```python
from build123d import *

# Parameters (mm, degrees)
SASE_TABAN1_W               = 80
SASE_TABAN1_H               = 130
Y_KSEKLIK_EKSTR_ZYON4_DEPTH = 3
SASE_TABAN1_5_W             = 86
SASE_TABAN1_5_H             = 136
SASE_TABAN1_5_W_2           = 80
SASE_TABAN1_5_H_2           = 130
Y_KSEKLIK_EKSTR_ZYON5_DEPTH = 10
Y_KSEKLIK_EKSTR_ZYON6_REACH = 138.755
KES_EKSTR_ZYON1_START       = -13
EKLEM_ORTA_W                = 36
EKLEM_ORTA_H                = 15
KES_EKSTR_ZYON1_DEPTH       = 13
KES_EKSTR_ZYON3_DEPTH       = 42
KES_EKSTR_ZYON4_START       = -6
KES_EKSTR_ZYON4_DEPTH       = 6
Y_KSEKLIK_EKSTR_ZYON7_START = -3
Y_KSEKLIK_EKSTR_ZYON7_DEPTH = 3
Y_KSEKLIK_EKSTR_ZYON8_DEPTH = 3


with BuildPart() as part:
    # sase_taban1 → Yükseklik-Ekstrüzyon4 (new body)
    with BuildSketch(Plane.XY):
        with Locations((1.981566113, 37.857486255)):
            Rectangle(SASE_TABAN1_W, SASE_TABAN1_H)
    extrude(amount=-Y_KSEKLIK_EKSTR_ZYON4_DEPTH)

    # sase_taban1<5> → Yükseklik-Ekstrüzyon5 (add)
    with BuildSketch(Plane.XY):
        with Locations((1.981566113, 37.857486255)):
            Rectangle(SASE_TABAN1_5_W, SASE_TABAN1_5_H)
        with Locations((1.981566113, 37.857486255)):
            Rectangle(SASE_TABAN1_5_W_2, SASE_TABAN1_5_H_2, mode=Mode.SUBTRACT)
    extrude(amount=-Y_KSEKLIK_EKSTR_ZYON5_DEPTH)

    # Yükseklik-Ekstrüzyon6: up to this face of the body (flat: up to its plane)
    y_kseklik_ekstr_zyon6_end = Plane(part.part.faces().sort_by_distance((-41.018433887, 37.857486255, -5))[0])
    # sase_eklem1 → Yükseklik-Ekstrüzyon6 (add, up to the picked face)
    with BuildSketch(Plane(origin=(44.981566113, 0, 0), x_dir=(0, 0, -1), z_dir=(1, 0, 0)), mode=Mode.PRIVATE) as y_kseklik_ekstr_zyon6_sk1:
        with BuildLine():
            Line((18, 105.857486255), (0, 105.857486255))
            Line((0, 105.857486255), (0, 97.857486255))
            Line((0, 97.857486255), (10, 89.857486255))
            Line((10, 89.857486255), (18, 89.857486255))
            Line((18, 89.857486255), (18, 92.857486255))
            ThreePointArc((18, 92.857486255), (13, 97.857486255), (18, 102.857486255))
            Line((18, 102.857486255), (18, 105.857486255))
        make_face()
    y_kseklik_ekstr_zyon6_tool1 = split(extrude(y_kseklik_ekstr_zyon6_sk1.sketch, amount=-Y_KSEKLIK_EKSTR_ZYON6_REACH, mode=Mode.PRIVATE), bisect_by=y_kseklik_ekstr_zyon6_end, keep=Keep.BOTH, mode=Mode.PRIVATE)
    add(y_kseklik_ekstr_zyon6_tool1.solids().sort_by(Axis((44.981566, 98.87954, -8.791936), (-1, 0, 0)))[0])

    # eklem_orta → Kes-Ekstrüzyon1 (cut)
    with BuildSketch(Plane.XZ.offset(-89.857486255).offset(KES_EKSTR_ZYON1_START)):
        with Locations((1.981566113, -10.5)):
            Rectangle(EKLEM_ORTA_W, EKLEM_ORTA_H)
    extrude(amount=KES_EKSTR_ZYON1_DEPTH, mode=Mode.SUBTRACT)

    # eklem_kablo → Kes-Ekstrüzyon3 (cut)
    with BuildSketch(Plane.ZY.offset(-19.981566113)):
        with BuildLine():
            Line((-5, 93.857486255), (-8.123475238, 91.358706065))
            ThreePointArc((-8.123475238, 91.358706065), (-10.068499616, 94.506792744), (-13.669872981, 95.357486255))
            ThreePointArc((-13.669872981, 95.357486255), (-13, 97.857486255), (-13.669872981, 100.357486255))
            ThreePointArc((-13.669872981, 100.357486255), (-7.988742413, 98.903075741), (-5, 93.857486255))
        make_face()
    extrude(amount=KES_EKSTR_ZYON3_DEPTH, mode=Mode.SUBTRACT)

    # eklem_kablo<2> → Kes-Ekstrüzyon4 (cut)
    with BuildSketch(Plane.ZY.offset(-19.981566113).offset(KES_EKSTR_ZYON4_START)):
        with BuildLine():
            Line((-8.123475238, 91.358706065), (-5, 93.857486255))
            ThreePointArc((-5, 93.857486255), (-7.988742413, 98.903075741), (-13.669872981, 100.357486255))
            ThreePointArc((-13.669872981, 100.357486255), (-13, 97.857486255), (-13.669872981, 95.357486255))
            ThreePointArc((-13.669872981, 95.357486255), (-10.068499616, 94.506792744), (-8.123475238, 91.358706065))
        make_face()
    extrude(amount=KES_EKSTR_ZYON4_DEPTH, mode=Mode.SUBTRACT)

    # eklem_sag_kapak → Yükseklik-Ekstrüzyon7 (add)
    with BuildSketch(Plane.ZY.offset(41.018433887).offset(Y_KSEKLIK_EKSTR_ZYON7_START)):
        with BuildLine():
            Line((-18, 102.857486255), (-18, 92.857486255))
            ThreePointArc((-18, 92.857486255), (-13, 97.857486255), (-18, 102.857486255))
        make_face()
    extrude(amount=Y_KSEKLIK_EKSTR_ZYON7_DEPTH)

    # eklem_sol_kapak → Yükseklik-Ekstrüzyon8 (add)
    with BuildSketch(Plane(origin=(44.981566113, 0, 0), x_dir=(0, 0, -1), z_dir=(1, 0, 0))):
        with BuildLine():
            Line((18, 102.857486255), (18, 92.857486255))
            ThreePointArc((18, 92.857486255), (13, 97.857486255), (18, 102.857486255))
        make_face()
    extrude(amount=-Y_KSEKLIK_EKSTR_ZYON8_DEPTH)


solid = part.part
```
Can you work these out from the model? Positions are in its coordinate system, mm. A direction names the side the tool comes from. Round coordinates to 2 decimals unless told otherwise and drop trailing zeros. Loops run counter-clockwise (first coordinate to the right, second up) from the corner with the lowest first, then second, coordinate; pieces in that order, holes last. Notation, with made-up numbers: M -19.75,43.5 L 0.25,43.5 A25 ccw 0.25,72.5 Z; hole C 32,-23 d5. An arc over 180 degrees is marked long. Write item = value, one per line. Start each with the question number.
(1) If we mould it in two halves opening along Y, with no side actions, what happens to faces 1 (the face through (-28, 89.857, -14)), 2 (the face through (31.14, 92.7, -6.45)), 3 (the face through (2, -28, -10))? For each: released by +Y, released by -Y, zero draft, split by the parting line, or undercut.
(2) Which directions (+Z, -Z, +X, -X, +Y, -Y) give clear straight access to the entire face, cutting with the end or side of a thin tool? Please do faces 4 (the face through (44.982, 39, -5)), 5 (the face through (23.024, 94.538, -10.112)), 6 (the face through (-38.018, 98, -16)).
(3) Suppose I cut it at C-C on x = 27.5. Write out the boundary of the cut face in (y, z).
(4) Suppose I cut it at B-B on x = -7. Write out the boundary of the cut face in (y, z).
(5) I'm going to push flat-ended pins straight in: P1, Ø1.5, axis at x = -19, y = 30, coming from the -Z side; P2, Ø9, axis at x = 30.5, z = -16, coming from the -Y side. Where does each tip first touch, or does it pass through?
(6) Suppose I cut it at A-A on y = 55. Write out the boundary of the cut face in (x, z).
(7) I need wall thicknesses on line 1 along X through (y, z) = (75, -7.5); line 2 along X through (y, z) = (92, -12.5); line 3 along Y through (x, z) = (8, -4.25). Which ranges of each line are inside material? Lowest first, please.
(8) Suppose I cut it at D-D on y = 97.5. Write out the boundary of the cut face in (x, z), plus the area to 3 significant figures.
Answer block:
q1.face_1 = released by -Y
q1.face_2 = undercut
q1.face_3 = zero draft
q2.face_4 = +Z, -Z, +X, +Y, -Y
q2.face_5 = none
q2.face_6 = -Z
q3.outline = M -30.14,-10 L -27.14,-10 L -27.14,-3 L 95.46,-3 L 89.86,-10 L 89.86,-18 L 92.86,-18 A5 cw 102.86,-18 L 105.86,-18 L 105.86,0 L -30.14,0 Z
q4.outline = M -30.14,-10 L -27.14,-10 L -27.14,-3 L 102.86,-3 L 102.86,-18 L 105.86,-18 L 105.86,0 L -30.14,0 Z
q5.P1 = -3
q5.P2 = 89.86
q6.outline = M -41.02,-10 L -38.02,-10 L -38.02,-3 L 41.98,-3 L 41.98,-10 L 44.98,-10 L 44.98,0 L -41.02,0 Z
q7.line_1 = -41.02 to -38.02, 41.98 to 44.98
q7.line_2 = -41.02 to -16.02, 19.98 to 44.98
q7.line_3 = -30.14 to -27.14, 102.86 to 105.86
q8.outline = M -41.02,-18 L -38.02,-18 L -38.02,-13.01 L -22.02,-13.01 L -22.02,-6.56 L -16.02,-6.56 L -16.02,-3 L 19.98,-3 L 19.98,-6.56 L 25.98,-6.56 L 25.98,-13.01 L 41.98,-13.01 L 41.98,-18 L 44.98,-18 L 44.98,0 L -41.02,0 Z
q8.area = 711 mm²
